```python
from build123d import *

# Parameters (mm, degrees)
SKETCH_1_W                  = 50
SKETCH_1_H                  = 150
EXTRUDE_1_DEPTH             = 3
SKETCH_2_W                  = 25
SKETCH_2_H                  = 3
EXTRUDE_2_DEPTH             = 12
SKETCH_3_W                  = 25
SKETCH_3_H                  = 3
EXTRUDE_3_DEPTH             = 12
HOLE_WIZARD_3_0_3_1_D       = 3
HOLE_WIZARD_3_0_3_1_DEPTH   = 50.000025
HOLE_WIZARD_5_5_5_5_1_D     = 5.5
HOLE_WIZARD_12_0_12_1_D     = 12
HOLE_WIZARD_12_0_12_1_DEPTH = 15.000025
FILLET_1_R                  = 20


with BuildPart() as part:
    # ｽｹｯﾁ1 → ﾎﾞｽ - 押し出し1 (new body)
    with BuildSketch(Plane(origin=(0, 0, 0), x_dir=(0, -1, 0), z_dir=(-1, 0, 0))):
        with Locations((-25, 0)):
            Rectangle(SKETCH_1_W, SKETCH_1_H)
    extrude(amount=-EXTRUDE_1_DEPTH)

    # ｽｹｯﾁ2 → ﾎﾞｽ - 押し出し2 (add)
    with BuildSketch(Plane(origin=(3, 0, 0), x_dir=(0, 0, -1), z_dir=(1, 0, 0))):
        with Locations((-62.5, 1.5)):
            Rectangle(SKETCH_2_W, SKETCH_2_H)
    extrude(amount=EXTRUDE_2_DEPTH)

    # ｽｹｯﾁ3 → ﾎﾞｽ - 押し出し3 (add)
    with BuildSketch(Plane(origin=(3, 0, 0), x_dir=(0, 0, -1), z_dir=(1, 0, 0))):
        with Locations((62.5, 1.5)):
            Rectangle(SKETCH_3_W, SKETCH_3_H)
    extrude(amount=EXTRUDE_3_DEPTH)

    # Ø3.0 (3) 直径の穴1
    with Locations(Plane(origin=(0, 0, 0), x_dir=(-1, 0, 0), z_dir=(0, -1, 0))):
        with Locations((-10, -67), (-10, 67)):
            Hole(HOLE_WIZARD_3_0_3_1_D / 2, depth=HOLE_WIZARD_3_0_3_1_DEPTH)

    # Ø5.5 (5.5) 直径の穴1 (through all)
    with Locations(Plane(origin=(3, 0, 0), x_dir=(0, 0, -1), z_dir=(1, 0, 0))):
        with Locations((60, 41), (-60, 41), (-60, 25), (60, 25)):
            Hole(HOLE_WIZARD_5_5_5_5_1_D / 2)

    # Ø12.0 (12) 直径の穴1
    with Locations(Plane.ZY):
        with Locations((0, 28)):
            Hole(HOLE_WIZARD_12_0_12_1_D / 2, depth=HOLE_WIZARD_12_0_12_1_DEPTH)

    # ﾌｨﾚｯﾄ1
    fillet_1_edges = [part.edges().sort_by_distance(p)[0] for p in [
        (1.5, 50, -75),
        (1.5, 50, 75),
    ]]
    fillet(fillet_1_edges, radius=FILLET_1_R)


solid = part.part
```
CAD build for the part. Positions are in the model's coordinates, mm. A direction names the side the tool comes from. Give positions to 0.01 mm unless a question says otherwise; leave off trailing zeros. Loops run counter-clockwise (first coordinate to the right, second up) from the corner with the lowest first, then second, coordinate; pieces in that order, holes last. Notation, with made-up numbers: (-4.5, 56.5) - (30.5, 56.5) arc R12 ccw to (30.5, 64.5) - close; hole circle Ø7 at (-17.75, -29). An arc over 180 degrees is marked (long way). Put each result on its own line as item: value.
Q1. Slice it at B-B (x = 10). Give the cut face in (y, z).
Filled in:
outline: (0, -75) - (3, -75) - (3, -68.5) - (0, -68.5) - close; (0, -65.5) - (3, -65.5) - (3, -50) - (0, -50) - close; (0, 50) - (3, 50) - (3, 65.5) - (0, 65.5) - close; (0, 68.5) - (3, 68.5) - (3, 75) - (0, 75) - close
Q2. Slice it at C-C (y = 25). Give the cut face in (x, z).
Filled in:
outline: (0, -75) - (3, -75) - (3, -62.75) - (0, -62.75) - close; (0, -57.25) - (3, -57.25) - (3, -5.2) - (0, -5.2) - close; (0, 5.2) - (3, 5.2) - (3, 57.25) - (0, 57.25) - close; (0, 62.75) - (3, 62.75) - (3, 75) - (0, 75) - close
Q3. Slice it at A-A (z = 67). Give the cut face in (x, y), plus the area to 3 significant figures.
Filled in:
outline: (0, 0) - (8.5, 0) - (8.5, 3) - (3, 3) - (3, 46) - (0, 46) - close; (11.5, 0) - (15, 0) - (15, 3) - (11.5, 3) - close
area: 165 mm²
Q4. Tool access for faces 4 (the face through (1.521, 43.986, 69.297)), 5 (the face through (9, 1, 50)), 6 (the face through (9, 3, -62)): list every direction of +Z, -Z, +X, -X, +Y, -Y with a clear straight run to the whole face (end or side of a thin tool).
Filled in:
face 4: +Z, +X, -X, +Y
face 5: +X, +Y, -Y
face 6: +Z, -Z, +X, +Y
Q5. Flat gauge pins, fed straight in: pin 1 (2.5 mm diameter, centred on x = 10, z = 67, fed in from -Y); pin 2 (4 mm diameter, centred on y = 28.5, z = 16.5, fed in from +X); pin 3 (3.5 mm diameter, centred on x = 10, z = -67, fed in from +Y). Where does each tip first touch, or does it go through?
Filled in:
pin 1: passes through
pin 2: stops at x = 3
pin 3: stops at y = 3
Q6. Probe line 1 along Z through (x, y) = (10, 2.05); line 2 along Y through (x, z) = (1.1, 60); line 3 along X through (y, z) = (1.1, -67). List the from-to ranges inside material, lowest first.
Filled in:
line 1: z = -75 to -68.5, -65.5 to -50, 50 to 65.5, 68.5 to 75
line 2: y = 0 to 22.25, 27.75 to 38.25, 43.75 to 49.36
line 3: x = 0 to 8.5, 11.5 to 15
Q7. Mould opens along X. For faces 1 (the face through (15, 2, 63)), 2 (the face through (1, 50, -1)), 3 (the face through (10.806, 1.521, 65.735)) say: pulls with the +X half, pulls with the -X half, needs draft (parallel to the pull), parting line crosses it, or undercut.
Filled in:
face 1: pulls with the +X half
face 2: needs draft
face 3: undercut
Q8. Slice it at D-D (z = 0). Give the cut face in (x, y).
Filled in:
outline: (0, 0) - (3, 0) - (3, 22) - (0, 22) - close; (0, 34) - (3, 34) - (3, 50) - (0, 50) - close
